from build123d import *

# Parameters (mm, degrees)
F1_DEPTH       = 20
F2_R           = 5
F5_D           = 3.2
F5_CBORE_D     = 6
F5_CBORE_DEPTH = 3
F6_W           = 18
F6_H           = 7.5
F7_DEPTH       = 10
F8_SIZE        = 1


# Not quite as in the source:
# - a feature of the source that left no trace in its solid (it failed there, or was rolled back) is left out


with BuildPart() as f1:
    # F0 (on Front) → F1 (new body, symmetric)
    with BuildSketch(Plane.XZ):
        Polygon((-24, 4), (-24, 0), (-24, -6), (24, -6), (24, 0), (24, 4), (3.1, 4), (7.1, 0), (-7.1, 0), (-3.1, 4), align=None)
    extrude(amount=F1_DEPTH, both=True)

    # F2
    f2_edges = [f1.edges().sort_by_distance(p)[0] for p in [
        (-24, 20, -1),
        (24, 20, -1),
        (24, -20, -1),
        (-24, -20, -1),
    ]]
    fillet(f2_edges, radius=F2_R)

    # F5 (through all)
    with Locations(Plane.XY.offset(4)):
        with Locations((13, -10), (-13, -10), (13, 10), (-13, 10)):
            CounterBoreHole(F5_D / 2, F5_CBORE_D / 2, F5_CBORE_DEPTH)

    # F6 (on face) → F7 (join)
    with BuildSketch(Plane(origin=(0, 0, -6), x_dir=(1, 0, 0), z_dir=(0, 0, -1))):
        with Locations((0, -16.25)):
            Rectangle(F6_W, F6_H)
    extrude(amount=-F7_DEPTH)

    # F8
    f8_edges = [f1.edges().sort_by_distance(p)[0] for p in [
        (0, 20, 4),
        (-22.535534, 18.535534, 4),
        (-24, 0, 4),
        (-22.535534, -18.535534, 4),
        (-11.05, -20, 4),
        (11.05, -20, 4),
        (22.535534, -18.535534, 4),
        (24, 0, 4),
        (22.535534, 18.535534, 4),
    ]]
    chamfer(f8_edges, length=F8_SIZE)


solid = f1.part
Geometry check sheet. Reference: the model listing, model coordinates, mm. A direction names the side the tool comes from. Round coordinates to 2 decimals unless told otherwise and drop trailing zeros. Loops run counter-clockwise (first coordinate to the right, second up) from the corner with the lowest first, then second, coordinate; pieces in that order, holes last. Notation, with made-up numbers: (-40, -30.75) -> (-7, -30.75) arc R9 cw to (-7, -18.75) -> close; hole circle Ø8 at (73, -7). An arc over 180 degrees is marked (long way). Answer as a JSON object with one key per item and string values. Group by question number.
Item 1: Set-up check for faces 1 (the face through (-11.7, -11.3, 1)), 2 (the face through (5.1, -4, 2)), 3 (the face through (-23, 18, -2)): record each of +Z, -Z, +X, -X, +Y, -Y from which the full face is reachable in a straight line by a thin tool's end or side.
Item 2: Depth check by flat-ended pin: pin 1 Ø4 at (x, y) = (13, 10) entering from +Z; pin 2 Ø1.2 at (x, z) = (-0.5, 2.5) entering from -Y. Enter the tip coordinate at first touch or a pass-through.
Item 3: Release check for a two-part mould opening along Z. For faces 4 (the face through (0, -4, 0)), 5 (the face through (-21.996, -18.063, 3.715)), 6 (the face through (14.27, -10.97, -2.55)) record: pulls with the +Z half, pulls with the -Z half, needs draft (parallel to the pull), parting line crosses it, or undercut.
Item 4: Cross-section at A-A, the plane y = 10. Record the cut outline in (x, z).
Item 5: Thickness scan on line 1 along Y through (x, z) = (13, -0.25); line 2 along Y through (x, z) = (14, -4.5); line 3 along Z through (x, y) = (0.5, 9.5). Record the ranges inside material, lowest first.
Item 6: Cross-section at D-D, the plane y = -2. Record the cut outline in (x, z).
Item 7: Cross-section at C-C, the plane z = -4.5. Record the cut outline in (x, y).
Item 8: Cross-section at B-B, the plane x = 13. Record the cut outline in (y, z), plus the area to 3 significant figures.
Determined:
{
 "1": {"face 1": "+Z", "face 2": "-Y", "face 3": "+Z, -Z, -X, +Y"},
 "2": {"pin 1": "stops at z = 1", "pin 2": "stops at y = 12.5"},
 "3": {"face 4": "undercut", "face 5": "pulls with the +Z half", "face 6": "needs draft"},
 "4": {"outline": "(-24, -6) -> (-14.6, -6) -> (-14.6, 1) -> (-16, 1) -> (-16, 4) -> (-23, 4) -> (-24, 3) -> close; (-11.4, -6) -> (11.4, -6) -> (11.4, 1) -> (10, 1) -> (10, 4) -> (3.1, 4) -> (7.1, 0) -> (-7.1, 0) -> (-3.1, 4) -> (-10, 4) -> (-10, 1) -> (-11.4, 1) -> close; (14.6, -6) -> (24, -6) -> (24, 3) -> (23, 4) -> (16, 4) -> (16, 1) -> (14.6, 1) -> close"},
 "5": {"line 1": "y = -20 to -11.6, -8.4 to 8.4, 11.6 to 20", "line 2": "y = -20 to -11.25, -8.75 to 8.75, 11.25 to 20", "line 3": "z = -6 to 0"},
 "6": {"outline": "(-24, -6) -> (24, -6) -> (24, 3) -> (23, 4) -> (3.1, 4) -> (7.1, 0) -> (-7.1, 0) -> (-3.1, 4) -> (-23, 4) -> (-24, 3) -> close"},
 "7": {"outline": "(-24, -15) arc R5 ccw to (-19, -20) -> (19, -20) arc R5 ccw to (24, -15) -> (24, 15) arc R5 ccw to (19, 20) -> (-19, 20) arc R5 ccw to (-24, 15) -> close; hole circle Ø3.2 at (-13, -10); hole circle Ø3.2 at (-13, 10); hole circle Ø3.2 at (13, -10); hole circle Ø3.2 at (13, 10)"},
 "8": {"outline": "(-20, -6) -> (-11.6, -6) -> (-11.6, 1) -> (-13, 1) -> (-13, 4) -> (-19, 4) -> (-20, 3) -> close; (-8.4, -6) -> (8.4, -6) -> (8.4, 1) -> (7, 1) -> (7, 4) -> (-7, 4) -> (-7, 1) -> (-8.4, 1) -> close; (11.6, -6) -> (20, -6) -> (20, 3) -> (19, 4) -> (13, 4) -> (13, 1) -> (11.6, 1) -> close", "area": "318 mm²"}
}
